Geometry: final body of the model. Coordinates: model frame, mm. Round coordinates to 2 decimals unless told otherwise and drop trailing zeros. Loops run counter-clockwise (first coordinate to the right, second up) from the corner with the lowest first, then second, coordinate; pieces in that order, holes last. Notation, with made-up numbers: M 51.5,-8 L 76.5,-8 A17 ccw 76.5,23 Z; hole C 10.5,-25 d11. An arc over 180 degrees is marked long. Answer as a JSON object with one key per item and string values.
Autodesk Inventor part; units mm, degrees
ref_plane "YZ Plane" through (0, 0, 0) normal (1, 0, 0) x (0, 1, 0)
ref_plane "XZ Plane" through (0, 0, 0) normal (0, 1, 0) x (-1, 0, 0)
ref_plane "XY Plane" through (0, 0, 0) normal (0, 0, 1) x (1, 0, 0)
sketch "Sketch1" plane through (0, 0, 0) normal (0, 0, 1) x (1, 0, 0)
  arc A0 (0, -63.5) -> (63.5, 0) centre (0, 0) ccw
  line L0 (0, 0) -> (-177.8, 0)
  line L1 (0, -63.5) -> (-177.8, -63.5)
  line L2 (-177.8, 0) -> (-177.8, -63.5)
  line L3 (0, 0) -> (63.5, 0)
  dimension "d0" = 127
  dimension "d1" = 177.8
  dimension "d2" = 177.8
extrude "Extrusion1" add sketch "Sketch1" along normal blind 1.5875
fillet "Fillet1" radius 3.175 1 edges at (63.5, 0, 0.7937)
fillet "Fillet2" radius 3.175 1 edges at (-177.8, 0, 0.7937)
fillet "Fillet3" radius 3.175 1 edges at (-177.8, -63.5, 0.7937)
properties part number "Flaps"
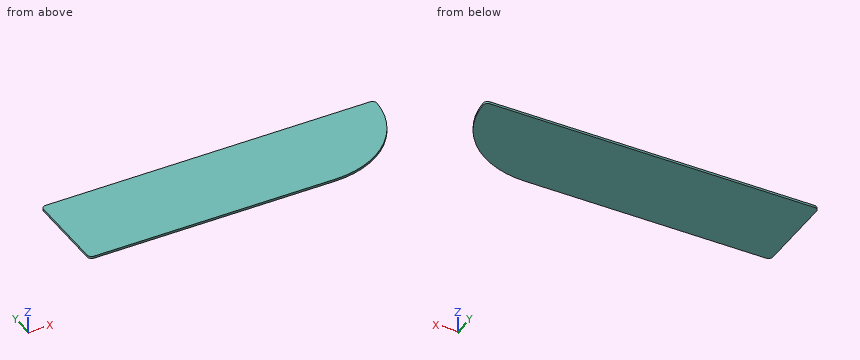
1) Cut plane A-A on z = 0.95. Return the cut outline in (x, y) (3 decimals).
Geometry results:
{"outline": "M -177.8,-60.325 A3.175 ccw -174.625,-63.5 L 0,-63.5 A63.5 ccw 63.412,-3.342 A3.175 ccw 60.241,0 L -174.625,0 A3.175 ccw -177.8,-3.175 Z"}
2) Cut plane B-B on y = -44. Return the cut outline in (x, z), and give its area (3 significant figures).
Geometry results:
{"outline": "M -177.8,0 L 45.78,0 L 45.78,1.59 L -177.8,1.59 Z", "area": "355 mm2"}
3) Cut plane C-C on x = 46.5. Return the cut outline in (y, z).
Geometry results:
{"outline": "M -43.24,0 L 0,0 L 0,1.59 L -43.24,1.59 Z"}
4) Line query: probe 1 along X at (y, z) = (-53.5, 1.45); probe 2 along Y at (x, z) = (44.5, 1); probe 3 along X at (y, z) = (-27, 0.1). Output: solid intervals per line, ascending.
Geometry results:
{"probe 1": "-177.8 to 34.21", "probe 2": "-45.3 to 0", "probe 3": "-177.8 to 57.47"}
